Here's how the part is built. I have some questions about the finished solid (model axes, mm). Face numbers are marked on the shaded views. A direction names the side the tool comes from. Coordinates: 2 decimals unless noted, no trailing zeros. Loops run counter-clockwise (first coordinate to the right, second up) from the corner with the lowest first, then second, coordinate; pieces in that order, holes last. Notation, with made-up numbers: (21.25, 17.5) -> (65.25, 17.5) arc R22 cw to (65.25, 33.5) -> close; hole circle Ø10 at (45.5, -6). An arc over 180 degrees is marked (long way). Answer as a JSON object with one key per item and string values. Group by question number.
Q1. I'm going to push flat-ended pins straight in: pin 1 (2 mm diameter, centred on y = 27.5, z = -3.5, fed in from -X); pin 2 (1 mm diameter, centred on x = 0.5, y = 28.5, fed in from +Z); pin 3 (0.9 mm diameter, centred on x = 0.5, z = 0, fed in from +Y); pin 4 (6 mm diameter, centred on y = 45, z = 3, fed in from -X). Where does each tip first touch, or does it pass through?
Q2. On a 3-axis mill with a long thin cutter (end or side, diameter ignored), from which of +Z, -Z, +X, -X, +Y, -Y can I reach the whole of each face in a straight line? I mean the marked faces 1 and 2. Say none if no direction works.
Q3. I want a section at B-B on y = 15. Write out the boundary of the cut face in (x, z).
Q4. I need wall thicknesses on line 1 (Z direction, x = -0.25, y = 20); line 2 (X direction, y = 36.5, z = 0); line 3 (Z direction, x = 2.5, y = 61). Which ranges of each line are inside material? Lowest first, please.
Q5. I want a section at A-A on x = 0. Write out the boundary of the cut face in (y, z).
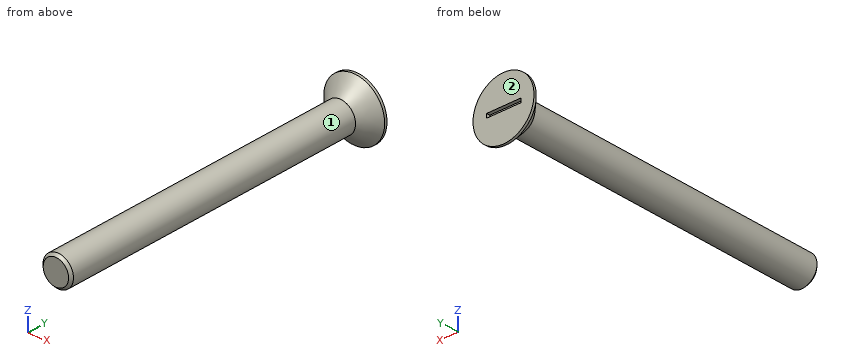
```python
from build123d import *

# Parameters (mm, degrees)
SKETCH_2_W          = 6.792543124
SKETCH_2_H          = 0.8
CUT_EXTRUDE_1_DEPTH = 0.7
CHAMFER_1_SIZE      = 0.5


with BuildPart() as part:
    # 草圖1 → 旋轉1 (revolve)
    with BuildSketch(Plane.XY):
        Polygon((0, 65), (6, 65), (6, 64.5), (3, 61.5), (3, 0), (0, 0), align=None)
    revolve(axis=Axis((0, -8.5328125, 0), (0, 1, 0)))

    # 草圖2 → 除料-伸長1 (cut)
    with BuildSketch(Plane(origin=(0, 65, 0), x_dir=(-1, 0, 0), z_dir=(0, 1, 0))):
        with Locations((0.075670859, 0)):
            Rectangle(SKETCH_2_W, SKETCH_2_H)
    extrude(amount=-CUT_EXTRUDE_1_DEPTH, mode=Mode.SUBTRACT)

    # 導角1
    chamfer_1_edges = [part.edges().sort_by_distance(p)[0] for p in [
        (-3, 0, 0),
    ]]
    chamfer(chamfer_1_edges, length=CHAMFER_1_SIZE)


solid = part.part
```
Result set:
{
 "1": {"pin 1": "stops at x = -1.66", "pin 2": "stops at z = 3", "pin 3": "stops at y = 65", "pin 4": "stops at x = -3"},
 "2": {"face 1": "-Y", "face 2": "+Z, -Z, +X, -X, +Y"},
 "3": {"outline": "circle Ø6 at (0, 0)"},
 "4": {"line 1": "z = -2.99 to 2.99", "line 2": "x = -3 to 3", "line 3": "z = -1.66 to 1.66"},
 "5": {"outline": "(0, -2.5) -> (0.5, -3) -> (61.5, -3) -> (64.5, -6) -> (65, -6) -> (65, -0.4) -> (64.3, -0.4) -> (64.3, 0.4) -> (65, 0.4) -> (65, 6) -> (64.5, 6) -> (61.5, 3) -> (0.5, 3) -> (0, 2.5) -> close"}
}
